```python
from build123d import *

# Parameters (mm, degrees)
SKETCH_1_R                      = 2.5
SKETCH_1_R_2                    = 3
EXTRUDE_1_DEPTH                 = 2.5
SKETCH_2_R                      = 2.45
SKETCH_2_R_2                    = 2.5
EXTRUDE_3_DEPTH                 = 8.6
CUT_EXTRUDE_1_REACH             = 53.724
SKETCH_2_2_R                    = 2.5
FILLET_1_R                      = 0.5
EXTRUDE_4_DEPTH                 = 8.6
FILLET_4_R                      = 1
CHAMFER_1_SIZE                  = 1
CUT_EXTRUDE_3_REACH             = 53.724
CUT_EXTRUDE_3_DIRECTION_2_DEPTH = 52.724136067
CHAMFER_2_SIZE                  = 1.5
CUT_EXTRUDE_5_REACH             = 53.724
CHAMFER_3_SIZE                  = 2
HOLE_WIZARD_M5_2_D              = 4.2
HOLE_WIZARD_M5_2_DEPTH          = 10
HOLE_WIZARD_M5_2_TIP            = 1.2618073
CUT_EXTRUDE_6_REACH             = 53.431
SKETCH_14_R                     = 2.5
CUT_EXTRUDE_7_DEPTH             = 52.431299391
CUT_EXTRUDE_7_DEPTH_BACK        = 52.431299391
SKETCH_15_W                     = 9
SKETCH_15_H                     = 44.55
SKETCH_15_W_2                   = 13.2
SKETCH_15_H_2                   = 52
SKETCH_17_R                     = 2.5
EXTRUDE_5_DEPTH                 = 3.5
FILLET_5_R                      = 2.4
SKETCH_18_W                     = 1.75
SKETCH_18_H                     = 52
EXTRUDE_6_DEPTH                 = 2
CHAMFER_4_SIZE                  = 1.5
SKETCH_19_R                     = 2
CUT_EXTRUDE_8_DEPTH             = 10


with BuildPart() as part:
    # 스케치1 → 보스-돌출1 (new body)
    with BuildSketch(Plane.XY):
        Polygon((-6.675534975, -27.705928987), (-2.173514753, -22.705928987), (13.286485247, -22.705928987), (18.839547821, -27.705928987), (41.669547821, -27.705928987), (41.669547821, 12.674071013), (30.011242494, 24.294071013), (14.761242494, 24.294071013), (9.469547821, 28.894071013), (0.269547821, 28.894071013), (-4.330452179, 24.294071013), (-27.130452179, 24.294071013), (-42.030452179, 9.394071013), (-42.030452179, -27.705928987), align=None)
        with Locations((-20.178757506, 7.504071013)):
            Circle(SKETCH_1_R, mode=Mode.SUBTRACT)
        with Locations((4.321242494, 23.004071013)):
            Circle(SKETCH_1_R, mode=Mode.SUBTRACT)
        with Locations((9.821242494, -1.495928987)):
            Circle(SKETCH_1_R_2, mode=Mode.SUBTRACT)
    extrude(amount=EXTRUDE_1_DEPTH)

    # 스케치2 → 보스-돌출3 (add)
    # profile 1 of 4: a face of its own
    with BuildSketch(Plane.XY.offset(2.5)):
        with Locations(Location((-5.130452179, 21.294071013, 0), (0, 0, 180))):
            Circle(SKETCH_2_R)
    # profile 2 of 4: a face of its own
    with BuildSketch(Plane.XY.offset(2.5)):
        with Locations(Location((-7.030452179, -23.705928987, 0), (0, 0, 180))):
            Circle(SKETCH_2_R)
    # profile 3 of 4: a face of its own
    with BuildSketch(Plane.XY.offset(2.5)):
        with BuildLine():
            Line((18.469547821, -14.205928987), (18.469547821, -27.37277949))
            Line((18.469547821, -27.37277949), (18.839547821, -27.705928987))
            Line((18.839547821, -27.705928987), (28.469547821, -27.705928987))
            Line((28.469547821, -27.705928987), (28.469547821, -14.205928987))
            Line((28.469547821, -14.205928987), (28.469547821, 24.294071013))
            Line((28.469547821, 24.294071013), (26.377590331, 24.294071013))
            Line((26.377590331, 24.294071013), (26.377590331, -10.138584797))
            ThreePointArc((26.377590331, -10.138584797), (21.182651731, -9.759570221), (18.469547821, -14.205928987))
        make_face()
        with Locations(Location((23.469547821, -14.205928987, 0), (0, 0, 180))):
            Circle(SKETCH_2_R_2, mode=Mode.SUBTRACT)
    # profile 4 of 4: a face of its own
    with BuildSketch(Plane.XY.offset(2.5)):
        with BuildLine():
            Line((-36.530452179, -2.705928987), (-36.530452179, -27.705928987))
            Line((-36.530452179, -27.705928987), (-29.030452179, -27.705928987))
            Line((-29.030452179, -27.705928987), (-29.030452179, -7.036056006))
            ThreePointArc((-29.030452179, -7.036056006), (-29.030452179, 1.624198032), (-36.530452179, -2.705928987))
        make_face()
        with Locations(Location((-31.530452179, -2.705928987, 0), (0, 0, 180))):
            Circle(SKETCH_2_R_2, mode=Mode.SUBTRACT)
    extrude(amount=EXTRUDE_3_DEPTH)

    # 스케치2<2> → 컷-돌출1 (cut, up to next)
    with BuildSketch(Plane.XY.offset(2.5), mode=Mode.PRIVATE) as cut_extrude_1_sk1:
        with Locations(Location((-31.530452179, -2.705928987, 0), (0, 0, 180))):
            Circle(SKETCH_2_2_R)
    cut_extrude_1_tool1 = extrude(cut_extrude_1_sk1.sketch, amount=-CUT_EXTRUDE_1_REACH, mode=Mode.PRIVATE) & part.part
    # 스케치2<2> → 컷-돌출1 (cut, up to next)
    with BuildSketch(Plane.XY.offset(2.5), mode=Mode.PRIVATE) as cut_extrude_1_sk2:
        with Locations(Location((23.469547821, -14.205928987, 0), (0, 0, 180))):
            Circle(SKETCH_2_2_R)
    cut_extrude_1_tool2 = extrude(cut_extrude_1_sk2.sketch, amount=-CUT_EXTRUDE_1_REACH, mode=Mode.PRIVATE) & part.part
    add(cut_extrude_1_tool1.solids().sort_by_distance((-31.530452, -2.705929, 2.5))[0], mode=Mode.SUBTRACT)
    add(cut_extrude_1_tool2.solids().sort_by_distance((23.469548, -14.205929, 2.5))[0], mode=Mode.SUBTRACT)

    # 필렛1
    fillet_1_edges = [part.edges().sort_by_distance(p)[0] for p in [
        (21.182651731, -9.759570221, 2.5),
        (-2.680452179, 21.294071013, 2.5),
        (-4.580452179, -23.705928987, 2.5),
        (18.469547821, -20.789354238, 2.5),
        (-36.530452179, -15.205928987, 2.5),
        (-29.030452179, -17.370992496, 2.5),
        (-29.030452179, 1.624198032, 2.5),
    ]]
    fillet(fillet_1_edges, radius=FILLET_1_R)

    # 스케치3 → 보스-돌출4 (add)
    with BuildSketch(Plane.XY.offset(2.5)):
        with BuildLine():
            Line((27.631077151, 8.755600344), (33.70801849, 8.755600344))
            ThreePointArc((33.70801849, 8.755600344), (34.415125271, 9.048493563), (34.70801849, 9.755600344))
            Line((34.70801849, 9.755600344), (34.70801849, 15.832541683))
            ThreePointArc((34.70801849, 15.832541683), (34.415125271, 16.539648464), (33.70801849, 16.832541683))
            Line((33.70801849, 16.832541683), (30.669547821, 16.832541683))
            ThreePointArc((30.669547821, 16.832541683), (27.813917825, 15.649701009), (26.631077151, 12.794071013))
            Line((26.631077151, 12.794071013), (26.631077151, 9.755600344))
            ThreePointArc((26.631077151, 9.755600344), (26.92397037, 9.048493563), (27.631077151, 8.755600344))
        make_face()
    extrude(amount=EXTRUDE_4_DEPTH)

    # 필렛4
    fillet_4_edges = [part.edges().sort_by_distance(p)[0] for p in [
        (29.522279368, 16.666153198, 2.5),
        (31.088783155, 8.755600344, 2.5),
        (32.188783155, 16.832541683, 2.5),
        (34.415125271, 9.048493563, 2.5),
        (34.70801849, 12.794071013, 2.5),
        (34.415125271, 16.539648464, 2.5),
    ]]
    fillet(fillet_4_edges, radius=FILLET_4_R)

    # 모따기1
    chamfer_1_edges = [part.edges().sort_by_distance(p)[0] for p in [
        (41.669547821, -27.705928987, 1.25),
        (-42.030452179, -27.705928987, 1.25),
    ]]
    chamfer(chamfer_1_edges, length=CHAMFER_1_SIZE)

    # 스케치8 → 컷-돌출3 (cut, up to next)
    with BuildSketch(Plane.XY.offset(2.5), mode=Mode.PRIVATE) as cut_extrude_3_sk1:
        Polygon((-15.730452179, 24.294071013), (-15.730452179, 16.844071013), (-34.580452179, 16.844071013), (-27.130452179, 24.294071013), align=None)
    cut_extrude_3_tool1 = extrude(cut_extrude_3_sk1.sketch, amount=-CUT_EXTRUDE_3_REACH, mode=Mode.PRIVATE) & part.part
    add(cut_extrude_3_tool1.solids().sort_by_distance((-23.445852, 20.263272, 2.5))[0], mode=Mode.SUBTRACT)

    # 스케치8 → 컷-돌출3 direction 2 (cut)
    with BuildSketch(Plane.XY.offset(2.5)):
        Polygon((-15.730452179, 24.294071013), (-15.730452179, 16.844071013), (-34.580452179, 16.844071013), (-27.130452179, 24.294071013), align=None)
    extrude(amount=CUT_EXTRUDE_3_DIRECTION_2_DEPTH, mode=Mode.SUBTRACT)

    # 모따기2
    chamfer_2_edges = [part.edges().sort_by_distance(p)[0] for p in [
        (-15.730452179, 16.844071013, 1.25),
        (-15.730452179, 24.294071013, 1.25),
    ]]
    chamfer(chamfer_2_edges, length=CHAMFER_2_SIZE)

    # 스케치10 → 컷-돌출5 (cut, up to next)
    with BuildSketch(Plane.XY.offset(2.5), mode=Mode.PRIVATE) as cut_extrude_5_sk1:
        Polygon((-37.030452179, -27.705928987), (-37.030452179, -2.705928987), (-37.030452179, 14.394071013), (-42.030452179, 9.394071013), (-42.030452179, -26.705928987), (-41.030452179, -27.705928987), align=None)
    cut_extrude_5_tool1 = extrude(cut_extrude_5_sk1.sketch, amount=-CUT_EXTRUDE_5_REACH, mode=Mode.PRIVATE) & part.part
    add(cut_extrude_5_tool1.solids().sort_by_distance((-39.472224, -7.830275, 2.5))[0], mode=Mode.SUBTRACT)

    # 모따기3
    chamfer_3_edges = [part.edges().sort_by_distance(p)[0] for p in [
        (-37.030452179, -27.705928987, 1.25),
    ]]
    chamfer(chamfer_3_edges, length=CHAMFER_3_SIZE)

    # M5 나사 구멍2
    with Locations(Plane(origin=(23.469547821, -27.705928987, 7.05), x_dir=(0, 0, -1), z_dir=(0, -1, 0))):
        with Locations((0, 0), (0, -56.25)):
            Hole(HOLE_WIZARD_M5_2_D / 2, depth=HOLE_WIZARD_M5_2_DEPTH)
            with Locations((0, 0, -(HOLE_WIZARD_M5_2_DEPTH + HOLE_WIZARD_M5_2_TIP / 2))):  # 118° drill point
                Cone(0, HOLE_WIZARD_M5_2_D / 2, HOLE_WIZARD_M5_2_TIP, mode=Mode.SUBTRACT)

    # 스케치14 → 컷-돌출6 (cut, up to next)
    with BuildSketch(Plane.XY.offset(2.5), mode=Mode.PRIVATE) as cut_extrude_6_sk1:
        with Locations((-10.530452179, -1.705928987)):
            Circle(SKETCH_14_R)
    cut_extrude_6_tool1 = extrude(cut_extrude_6_sk1.sketch, amount=-CUT_EXTRUDE_6_REACH, mode=Mode.PRIVATE) & part.part
    add(cut_extrude_6_tool1.solids().sort_by_distance((-10.530452, -1.705929, 2.5))[0], mode=Mode.SUBTRACT)

    # 스케치15 → 컷-돌출7 (cut, two sides: drawn at the far end of the back side and taken through both)
    with BuildSketch(Plane.XY.offset(2.5).offset(-CUT_EXTRUDE_7_DEPTH_BACK)):
        with Locations((-32.530452179, -5.430928987)):
            Rectangle(SKETCH_15_W, SKETCH_15_H)
        with Locations((35.069547821, -1.705928987)):
            Rectangle(SKETCH_15_W_2, SKETCH_15_H_2)
    extrude(amount=CUT_EXTRUDE_7_DEPTH + CUT_EXTRUDE_7_DEPTH_BACK, mode=Mode.SUBTRACT)

    # 스케치17 → 보스-돌출5 (add)
    with BuildSketch(Plane.ZY.offset(-26.377590331)):
        with Locations(Location((6.5, 13.294071013, 0), (0, 0, 180))):
            Circle(SKETCH_17_R)
    extrude(amount=EXTRUDE_5_DEPTH)

    # 필렛5
    fillet_5_edges = [part.edges().sort_by_distance(p)[0] for p in [
        (22.877590331, 13.294071013, 9),
    ]]
    fillet(fillet_5_edges, radius=FILLET_5_R)

    # 스케치18 → 보스-돌출6 (add)
    with BuildSketch(Plane.XY.offset(11.1)):
        with Locations((27.594547821, -1.705928987)):
            Rectangle(SKETCH_18_W, SKETCH_18_H)
    extrude(amount=EXTRUDE_6_DEPTH)

    # 모따기4
    chamfer_4_edges = [part.edges().sort_by_distance(p)[0] for p in [
        (-28.030452179, -27.705928987, 1.25),
        (-28.030452179, 16.844071013, 1.25),
        (28.469547821, 24.294071013, 6.55),
        (28.469547821, -27.705928987, 6.55),
    ]]
    chamfer(chamfer_4_edges, length=CHAMFER_4_SIZE)

    # 스케치19 → 컷-돌출8 (cut)
    with BuildSketch(Plane.XY.offset(2.5)):
        with Locations((-10.200452179, 20.994071013)):
            Circle(SKETCH_19_R)
    extrude(amount=-CUT_EXTRUDE_8_DEPTH, mode=Mode.SUBTRACT)


solid = part.part
```
For this review, take the finished solid that the model builds, in its own axes (mm). A direction names the side the tool comes from. Round coordinates to 2 decimals unless told otherwise and drop trailing zeros. Write each loop counter-clockwise with the first axis right and the second up, starting at its lowest first coordinate (ties: lowest second). Pieces come first, ordered by that corner, then holes. Notation, with made-up numbers: (33, 57) - (85, 57) arc R25 cw to (85, 74) - close; hole circle Ø5 at (78, -39). An arc over 180 degrees is marked (long way). Use CSV: the item, a comma, the result in double quotes.
1) Add section A-A on y = 3.5. Write out the cut boundary in (x, z).
Conclusion:
outline,"(-28.03, 0) - (28.47, 0) - (28.47, 13.1) - (26.72, 13.1) - (26.72, 11.1) - (26.38, 11.1) - (26.38, 2.5) - (-28.03, 2.5) - close"
2) Add section C-C on z = 1. Write out the cut boundary in (x, y).
Conclusion:
outline,"(-28.03, -26.21) - (-26.53, -27.71) - (-6.68, -27.71) - (-2.17, -22.71) - (13.29, -22.71) - (18.84, -27.71) - (26.97, -27.71) - (28.47, -26.21) - (28.47, 22.79) - (26.97, 24.29) - (14.76, 24.29) - (9.47, 28.89) - (0.27, 28.89) - (-4.33, 24.29) - (-14.23, 24.29) - (-15.73, 22.79) - (-15.73, 18.34) - (-17.23, 16.84) - (-26.53, 16.84) - (-28.03, 15.34) - close; hole circle Ø5 at (-20.18, 7.5); hole circle Ø5 at (-10.53, -1.71); hole circle Ø4 at (-10.2, 20.99); hole circle Ø5 at (4.32, 23); hole circle Ø6 at (9.82, -1.5); hole circle Ø5 at (23.47, -14.21)"
3) Wall thickness on line 1 along X through (y, z) = (-3, 9); line 2 along X through (y, z) = (-14, 6); line 3 along X through (y, z) = (0, 1.5): over which ranges is each line inside the solid? List them lowest first. Write a range as from..to.
Conclusion:
line 1,"x = -28.03..-26.54, 26.38..28.47"
line 2,"x = 18.47..20.98, 25.96..28.47"
line 3,"x = -28.03..-12.36, -8.7..7.22, 12.42..28.47"
4) For faces 5 (the flat face through (5, 28.894, 1)), 6 (the flat face through (5, -22.706, 1)), 7 (the flat face through (-5, 21, 11.1)), 8 (the cylindrical face through (-6.712, -26.135, 6.993)), 9 (the flat face through (-22, 16.844, 1)), list the 3-axis set-ups (+Z, -Z, +X, -X, +Y, -Y) from which the entire face can be reached by the end or side of a thin tool; tool diameter is ignored.
Conclusion:
face 5,"+Z, -Z, +X, -X, +Y"
face 6,"+Z, -Z, -Y"
face 7,"+Z, -X, +Y, -Y"
face 8,"+Z"
face 9,"+Z, -Z, -X, +Y"
5) The part is to be moulded in two halves that separate along X. For faces 1 (the cylindrical face through (25.84, 14.25, 4.19)), 2 (the cylindrical face through (-11.79, 19.78, 1.27)), 3 (the cylindrical face through (5.67, 25.11, 1.23)), 4 (the flat face through (-27.291, -26.945, 1.233)), say which applies: pulls with the +X half, pulls with the -X half, needs draft (parallel to the pull), parting line crosses it, or undercut.
Conclusion:
face 1,"needs draft"
face 2,"undercut"
face 3,"undercut"
face 4,"pulls with the -X half"
6) Clearance check with flat-ended pins moving along their axes: pin 1 Ø6 at (x, z) = (-1, 7) entering from -Y; pin 2 Ø3 at (x, z) = (-10, 1.5) entering from +Y; pin 3 Ø4 at (x, y) = (-16, -12) entering from +Z; pin 4 Ø3.5 at (x, y) = (-10.2, 20.99) entering from +Z. State where each tip first meets the part, or that it passes through.
Conclusion:
pin 1,"stops at y = 19.12"
pin 2,"stops at y = 24.29"
pin 3,"stops at z = 2.5"
pin 4,"passes through"
7) Add section B-B on x = 6. Write out the cut boundary in (y, z), and give its area (3 significant figures).
Conclusion:
outline,"(-22.71, 0) - (21.15, 0) - (21.15, 2.5) - (-22.71, 2.5) - close; (24.86, 0) - (28.89, 0) - (28.89, 2.5) - (24.86, 2.5) - close"
area,"120 mm^2"
